Answer from the drawing. Dimensions are ordinates in mm from the lowest x, y and z of the part. Give positions to 0.01 mm unless a question says otherwise; leave off trailing zeros. Order: outer loops, then holes, each group sorted by start corner. A loop starts at its lowest first (then second) coordinate and runs counter-clockwise, first axis right, second up. Notation, with made-up numbers: (46, -13.5) -> (71, -13.5) arc R25 ccw to (71, 16.5) -> close; hole circle Ø1 at (47, 66). An arc over 180 degrees is marked (long way). Answer as CSV lines item,"result". Start each with the question number.
1) Find section C-C (z = 38). Determine the outline of the cut face in (x, y), and give its area (3 significant figures).
2) Find section D-D (y = 11). Determine the outline of the cut face in (x, z), and give its area (3 significant figures).
3) Straight lines are drawn through the part: L1, parallel to X at y = 11.75, z = 38; L2, parallel to X at y = 3.75, z = 38; L3, parallel to X at y = 10, z = 37.5 (1 decimal). For each, find the intervals that lie inside material, in ascending order. Write a range as from..to.
4) Find section A-A (y = 4.75). Determine the outline of the cut face in (x, z), and give its area (3 significant figures).
5) The mould has two halves that part along X. Classify the marked faces 1, 2 and 3: +X half, -X half, draft (parallel to the pull), parting line (faces both ways), or undercut.
6) Flat-ended cylindrical pins translate along their axes: pin 1 Ø2.5 at (x, z) = (4.5, 4) entering from -Y; pin 2 Ø1.7 at (x, y) = (23.5, 12.5) entering from +Z; pin 3 Ø1.3 at (x, z) = (32, 1) entering from +Y; pin 4 Ø4 at (x, z) = (35, 40) entering from +Y. Find the tip coordinate at first contact, or state that the pin passes through.
7) Find section B-B (x = 53.5). Determine the outline of the cut face in (y, z).
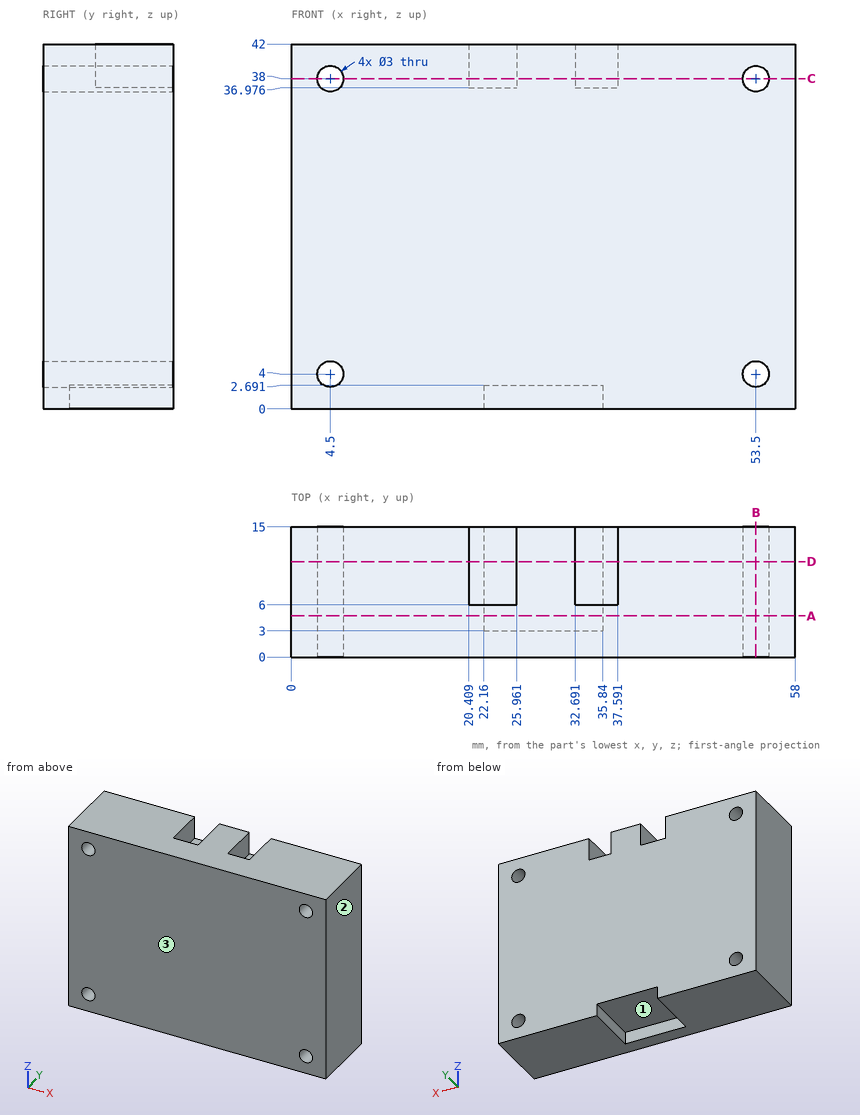
Findings below:
1,outline,"(0, 0) -> (3, 0) -> (3, 15) -> (0, 15) -> close; (6, 0) -> (52, 0) -> (52, 15) -> (37.59, 15) -> (37.59, 6) -> (32.69, 6) -> (32.69, 15) -> (25.96, 15) -> (25.96, 6) -> (20.41, 6) -> (20.41, 15) -> (6, 15) -> close; (55, 0) -> (58, 0) -> (58, 15) -> (55, 15) -> close"
1,area,"686 mm²"
2,outline,"(0, 0) -> (22.16, 0) -> (22.16, 2.69) -> (35.84, 2.69) -> (35.84, 0) -> (58, 0) -> (58, 42) -> (37.59, 42) -> (37.59, 36.98) -> (32.69, 36.98) -> (32.69, 42) -> (25.96, 42) -> (25.96, 36.98) -> (20.41, 36.98) -> (20.41, 42) -> (0, 42) -> close; hole circle Ø3 at (4.5, 4); hole circle Ø3 at (4.5, 38); hole circle Ø3 at (53.5, 4); hole circle Ø3 at (53.5, 38)"
2,area,"2,320 mm²"
3,L1,"0..3, 6..20.41, 25.96..32.69, 37.59..52, 55..58"
3,L2,"0..3, 6..52, 55..58"
3,L3,"0..3.1, 5.9..20.4, 26..32.7, 37.6..52.1, 54.9..58"
4,outline,"(0, 0) -> (22.16, 0) -> (22.16, 2.69) -> (35.84, 2.69) -> (35.84, 0) -> (58, 0) -> (58, 42) -> (0, 42) -> close; hole circle Ø3 at (4.5, 4); hole circle Ø3 at (4.5, 38); hole circle Ø3 at (53.5, 4); hole circle Ø3 at (53.5, 38)"
4,area,"2,370 mm²"
5,face 1,"undercut"
5,face 2,"+X half"
5,face 3,"draft"
6,pin 1,"through"
6,pin 2,"z = 36.98"
6,pin 3,"y = 3"
6,pin 4,"y = 6"
7,outline,"(0, 0) -> (15, 0) -> (15, 2.5) -> (0, 2.5) -> close; (0, 5.5) -> (15, 5.5) -> (15, 36.5) -> (0, 36.5) -> close; (0, 39.5) -> (15, 39.5) -> (15, 42) -> (0, 42) -> close"
